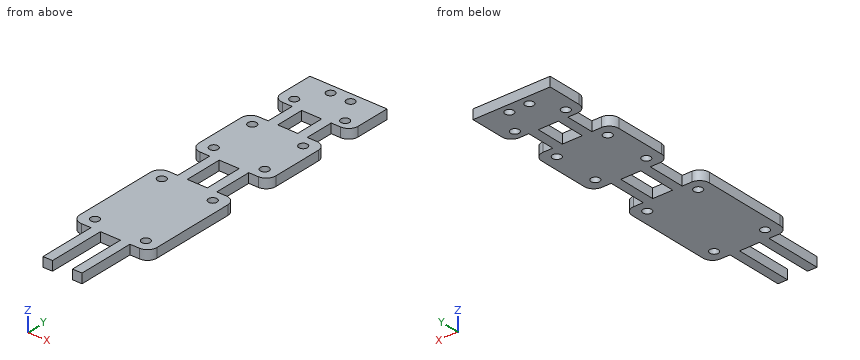
from build123d import *

# Parameters (mm, degrees)
SKETCH1_R           = 0.9
SKETCH1_W           = 4.2
SKETCH1_H           = 6
SKETCH1_H_2         = 8
BOSS_EXTRUDE1_DEPTH = 2


with BuildPart() as part:
    # Sketch1 → Boss-Extrude1 (new body)
    with BuildSketch(Plane.XY):
        with BuildLine():
            Line((2, 47.74), (4, 47.74))
            Line((4, 47.74), (4, 55.74))
            Line((4, 55.74), (2, 55.74))
            ThreePointArc((2, 55.74), (0.585786438, 56.325786438), (0, 57.74))
            Line((0, 57.74), (0, 68.385))
            ThreePointArc((0, 68.385), (0.585786438, 69.799213562), (2, 70.385))
            Line((2, 70.385), (4, 70.385))
            Line((4, 70.385), (4, 76.385))
            Line((4, 76.385), (2, 76.385))
            ThreePointArc((2, 76.385), (0.585786438, 76.970786438), (0, 78.385))
            Line((0, 78.385), (0, 85.59))
            Line((0, 85.59), (16.2, 85.59))
            Line((16.2, 85.59), (16.2, 78.385))
            ThreePointArc((16.2, 78.385), (15.614213562, 76.970786438), (14.2, 76.385))
            Line((14.2, 76.385), (12.2, 76.385))
            Line((12.2, 76.385), (12.2, 70.385))
            Line((12.2, 70.385), (14.2, 70.385))
            ThreePointArc((14.2, 70.385), (15.614213562, 69.799213562), (16.2, 68.385))
            Line((16.2, 68.385), (16.2, 57.74))
            ThreePointArc((16.2, 57.74), (15.614213562, 56.325786438), (14.2, 55.74))
            Line((14.2, 55.74), (12.2, 55.74))
            Line((12.2, 55.74), (12.2, 47.74))
            Line((12.2, 47.74), (14.2, 47.74))
            ThreePointArc((14.2, 47.74), (15.614213562, 47.154213562), (16.2, 45.74))
            Line((16.2, 45.74), (16.2, 28))
            ThreePointArc((16.2, 28), (15.614213562, 26.585786438), (14.2, 26))
            Line((14.2, 26), (12.2, 26))
            Line((12.2, 26), (12.2, 14))
            Line((12.2, 14), (10.2, 14))
            Line((10.2, 14), (10.2, 26))
            Line((10.2, 26), (6, 26))
            Line((6, 26), (6, 14))
            Line((6, 14), (4, 14))
            Line((4, 14), (4, 26))
            Line((4, 26), (2, 26))
            ThreePointArc((2, 26), (0.585786438, 26.585786438), (0, 28))
            Line((0, 28), (0, 45.74))
            ThreePointArc((0, 45.74), (0.585786438, 47.154213562), (2, 47.74))
        make_face()
        with Locations((13.45, 45.24)):
            Circle(SKETCH1_R, mode=Mode.SUBTRACT)
        with Locations((2.75, 67.885)):
            Circle(SKETCH1_R, mode=Mode.SUBTRACT)
        with Locations((13.45, 58.24)):
            Circle(SKETCH1_R, mode=Mode.SUBTRACT)
        with Locations((13.45, 78.385)):
            Circle(SKETCH1_R, mode=Mode.SUBTRACT)
        with Locations((2.75, 28.5)):
            Circle(SKETCH1_R, mode=Mode.SUBTRACT)
        with Locations((2.75, 78.385)):
            Circle(SKETCH1_R, mode=Mode.SUBTRACT)
        with Locations((2.75, 58.24)):
            Circle(SKETCH1_R, mode=Mode.SUBTRACT)
        with Locations((6, 83.635)):
            Circle(SKETCH1_R, mode=Mode.SUBTRACT)
        with Locations((13.45, 28.5)):
            Circle(SKETCH1_R, mode=Mode.SUBTRACT)
        with Locations((13.45, 67.885)):
            Circle(SKETCH1_R, mode=Mode.SUBTRACT)
        with Locations((10.2, 83.635)):
            Circle(SKETCH1_R, mode=Mode.SUBTRACT)
        with Locations((2.75, 45.24)):
            Circle(SKETCH1_R, mode=Mode.SUBTRACT)
        with Locations((8.1, 73.385)):
            Rectangle(SKETCH1_W, SKETCH1_H, mode=Mode.SUBTRACT)
        with Locations((8.1, 51.74)):
            Rectangle(SKETCH1_W, SKETCH1_H_2, mode=Mode.SUBTRACT)
    extrude(amount=BOSS_EXTRUDE1_DEPTH)


solid = part.part
Here's how the part is built. I have some questions about the finished solid (model axes, mm). Round coordinates to 2 decimals unless told otherwise and drop trailing zeros. Write each loop counter-clockwise with the first axis right and the second up, starting at its lowest first coordinate (ties: lowest second). Pieces come first, ordered by that corner, then holes. Notation, with made-up numbers: (40.5, -36.75) -> (50.5, -36.75) arc R20 cw to (50.5, -4.75) -> close; hole circle Ø8 at (55, 18.5). An arc over 180 degrees is marked (long way). One line per item, written item: value.
1) If I drill on line 1 (X direction, y = 45.24, z = 0.9); line 2 (Y direction, x = 3.75, z = 1.3) (3 decimals); line 3 (X direction, y = 70.5, z = 0.2), over which ranges is the centre line in solid material (lowest first)? Write a range as [from, to].
Filled sheet:
line 1: x = [0, 1.85], [3.65, 12.55], [14.35, 16.2]
line 2: y = [26, 47.74], [55.74, 70.385], [76.385, 85.59]
line 3: x = [4, 6], [10.2, 12.2]
2) I'm going to push flat-ended pins straight in: pin 1 Ø1 at (y, z) = (51.5, 1) entering from -X; pin 2 Ø1 at (x, z) = (3, 1.5) entering from -Y; pin 3 Ø4 at (x, y) = (12.5, 57.5) entering from -Z; pin 4 Ø1 at (y, z) = (70, 1) entering from -X. Where does each tip first touch, or does it pass through?
Filled sheet:
pin 1: stops at x = 4
pin 2: stops at y = 26
pin 3: stops at z = 0
pin 4: stops at x = 0.34
3) Suppose I cut it at B-B on z = 1.35. Give the number of separate pieces and of enclosed holes in the cut face, plus the area to 3 significant figures.
Filled sheet:
separate pieces: 1
enclosed holes: 14
area: 803 mm2
4) Suppose I cut it at A-A on y = 19.5. List the corners of the cut face in (x, z) for me, plus the area to 3 significant figures.
Filled sheet:
outline: (4, 0) -> (6, 0) -> (6, 2) -> (4, 2) -> close; (10.2, 0) -> (12.2, 0) -> (12.2, 2) -> (10.2, 2) -> close
area: 8.00 mm2
